Check sheet for the modelled part. Datum: model origin and axes. Units: mm. A direction names the side the tool comes from. Coordinates: 2 decimals unless noted, no trailing zeros. Loops run counter-clockwise (first coordinate to the right, second up) from the corner with the lowest first, then second, coordinate; pieces in that order, holes last. Notation, with made-up numbers: (1, -23) - (52, -23) arc R12 ccw to (52, -9) - close; hole circle Ø5 at (78.25, 78.5). An arc over 180 degrees is marked (long way). Write each question's results on one line, items separated by ' | '. Start each with the question number.
1. Draft check along Z on faces 1 (the face through (0, -13.2, -2.3)), 2 (the face through (0, 3.5, -0.1)), 3 (the face through (-0.01, 0.07, 1.5)). Enter one of: released by +Z, released by -Z, zero draft, split by the parting line, or undercut.
2. Cross-section at B-B (x = -0.5). Record the cut outline in (y, z).
3. Cross-section at C-C (y = 0.5). Record the cut outline in (x, z), and give its area (3 significant figures).
4. Cross-section at D-D (y = -13). Record the cut outline in (x, z).
5. Thickness scan on line 1 (Y direction, x = 0.1, z = 0); line 2 (X direction, y = -2.25, z = -3); line 3 (Y direction, x = 0.25, z = -0.75). Record the ranges inside material, lowest first. Write a range as [from, to].
6. Gauge pin test, flat ends, axial feed: P1, Ø2, axis at x = -2.5, y = -8, coming from the -Z side; P2, Ø2.5, axis at x = -2.5, y = -14.5, coming from the +Z side; P3, Ø1, axis at x = -3.5, z = -0.5, coming from the +Y side. Record the tip position at first contact, or that the pin passes through.
7. Cross-section at A-A (z = 0). Record the cut outline in (x, y), and give its area (3 significant figures).
8. Tool access check on faces 4 (the face through (-4, -12, 0)), 5 (the face through (1.5, -12, 0)), 6 (the face through (0, -6, 3.5)). Record the directions out of +Z, -Z, +X, -X, +Y, -Y that give a thin tool (end or side, any length) a straight path to the whole face; none if there is none.
```python
from build123d import *

# Parameters (mm, degrees)
SKETCH1_R           = 1.5
BOSS_EXTRUDE1_DEPTH = 1
SKETCH2_W           = 8
SKETCH2_H           = 8
BOSS_EXTRUDE2_DEPTH = 1
BOSS_EXTRUDE3_DEPTH = 1


with BuildPart() as part:
    # Sketch1 → Boss-Extrude1 (new, symmetric)
    with BuildSketch(Plane(origin=(0, 0, 0), x_dir=(0, 0, -1), z_dir=(1, 0, 0))):
        with BuildLine():
            Line((-3.5, 0), (-3.5, -12))
            Line((-3.5, -12), (3.5, -12))
            Line((3.5, -12), (3.5, 0))
            ThreePointArc((3.5, 0), (0, 3.5), (-3.5, 0))
        make_face()
        Circle(SKETCH1_R, mode=Mode.SUBTRACT)
    extrude(amount=BOSS_EXTRUDE1_DEPTH, both=True)

    # Sketch2 → Boss-Extrude2 (add, symmetric)
    with BuildSketch(Plane.XY):
        with Locations((-2, -16)):
            Rectangle(SKETCH2_W, SKETCH2_H)
    extrude(amount=BOSS_EXTRUDE2_DEPTH, both=True)

    # Sketch3 → Boss-Extrude3 (add, symmetric)
    with BuildSketch(Plane(origin=(0, 0, 0), x_dir=(0, 0, -1), z_dir=(1, 0, 0))):
        Polygon((-3.5, -12), (-1, -14.5), (-1, -12), align=None)
        Polygon((1, -12), (3.5, -12), (1, -14.5), align=None)
    extrude(amount=BOSS_EXTRUDE3_DEPTH, both=True)


solid = part.part
```
Established:
1) face 1: released by -Z | face 2: split by the parting line | face 3: undercut
2) outline: (-20, -1) - (-14.5, -1) - (-12, -3.5) - (0, -3.5) arc R3.5 ccw to (0, 3.5) - (-12, 3.5) - (-14.5, 1) - (-20, 1) - close; hole circle Ø3 at (0, 0)
3) outline: (-1, -3.46) - (1, -3.46) - (1, -1.41) - (-1, -1.41) - close; (-1, 1.41) - (1, 1.41) - (1, 3.46) - (-1, 3.46) - close | area: 8.20 mm^2
4) outline: (-6, -1) - (-1, -1) - (-1, -2.5) - (1, -2.5) - (1, -1) - (2, -1) - (2, 1) - (1, 1) - (1, 2.5) - (-1, 2.5) - (-1, 1) - (-6, 1) - close
5) line 1: [-20, -1.5], [1.5, 3.5] | line 2: [-1, 1] | line 3: [-20, -1.3], [1.3, 3.42]
6) P1: through | P2: z = 1 | P3: y = -12
7) outline: (-6, -20) - (2, -20) - (2, -12) - (1, -12) - (1, -1.5) - (-1, -1.5) - (-1, -12) - (-6, -12) - close; (-1, 1.5) - (1, 1.5) - (1, 3.5) - (-1, 3.5) - close | area: 89.0 mm^2
8) face 4: +Z, -Z, -X, +Y | face 5: +Z, -Z, +X, +Y | face 6: +Z, +X, -X, +Y, -Y
